Check sheet for the modelled part. Datum: model origin and axes. Units: mm. A direction names the side the tool comes from. Round coordinates to 2 decimals unless told otherwise and drop trailing zeros. Order: outer loops, then holes, each group sorted by start corner. A loop starts at its lowest first (then second) coordinate and runs counter-clockwise, first axis right, second up.
from build123d import *

# Parameters (mm, degrees)
SKETCH_1_R          = 14
SKETCH_1_R_2        = 7.5
EXTRUDE_1_DEPTH     = 35
SKETCH_2_R          = 7.5
CUT_EXTRUDE_1_DEPTH = 35
SKETCH_3_R          = 2.5
EXTRUDE_2_DEPTH     = 14
SKETCH_3_2_R        = 2.5
CUT_EXTRUDE_2_DEPTH = 3


with BuildPart() as part:
    # Sketch 1 → Extrude 1 (new body)
    with BuildSketch(Plane(origin=(0, 0, 0), x_dir=(1, 0, 0), z_dir=(0, 1, 0))):
        with Locations(Location((35, 0, 0), (0, 0, 270))):
            Circle(SKETCH_1_R)
        with Locations(Location((35, 0, 0), (0, 0, 270))):
            Circle(SKETCH_1_R_2, mode=Mode.SUBTRACT)
    extrude(amount=EXTRUDE_1_DEPTH)

    # Sketch 2 → Cut-Extrude 1 (cut)
    with BuildSketch(Plane.XY):
        with Locations(Location((35, 20, 0), (0, 0, 180))):
            Circle(SKETCH_2_R)
    extrude(amount=CUT_EXTRUDE_1_DEPTH, mode=Mode.SUBTRACT)

    # Sketch 3 → Extrude 2 (add)
    with BuildSketch(Plane.XY):
        Polygon((0, 0), (35, 0), (35, -7), (15, -7), (15, -18), (0, -18), align=None)
        with Locations((7, -13)):
            Circle(SKETCH_3_R, mode=Mode.SUBTRACT)
    extrude(amount=EXTRUDE_2_DEPTH)

    # Sketch 3_2 → Cut-Extrude 2 (cut)
    with BuildSketch(Plane.XY):
        Polygon((0, 0), (35, 0), (35, -7), (15, -7), (15, -18), (0, -18), align=None)
        with Locations((7, -13)):
            Circle(SKETCH_3_2_R, mode=Mode.SUBTRACT)
    extrude(amount=CUT_EXTRUDE_2_DEPTH, mode=Mode.SUBTRACT)


solid = part.part
1) Scan lines: line 1 (Y direction, x = 7, z = 9); line 2 (X direction, y = 12, z = 0); line 3 (Z direction, x = 5, y = -3). Record each from-to range of solid material in increasing order.
2) Sectioned sample at C-C on y = -13. Record the cut outline in (x, z), and give its area (3 significant figures).
3) Gauge pin test, flat ends, axial feed: pin 1 (2 mm diameter, centred on x = 32, z = 5, fed in from +Y); pin 2 (6 mm diameter, centred on y = 4.5, z = -3.5, fed in from +X); pin 3 (2 mm diameter, centred on x = 42, y = 24.5, fed in from +Z). Record the tip position at first contact, or that the pin passes through.
4) Sectioned sample at B-B on z = 3.75. Record the cut outline in (x, y).
5) Set-up check for faces 4 (the face through (13, 0, 8)), 5 (the face through (41, 0, -6)), 6 (the face through (35.33, 17.255, -7.493)): record each of +Z, -Z, +X, -X, +Y, -Y from which the full face is reachable in a straight line by a thin tool's end or side.
6) Sectioned sample at A-A on x = 8.5. Record the cut outline in (y, z), and give its area (3 significant figures).
7) Draft check along Z on faces 1 (the face through (35, -3, 8)), 2 (the face through (35.616, 17.255, -13.986)), 3 (the face through (32, 0, 5)). Enter one of: pulls with the +Z half, pulls with the -Z half, needs draft (parallel to the pull), parting line crosses it, or undercut.
8) Sectioned sample at D-D on z = 8.75. Record the cut outline in (x, y), and give its area (3 significant figures).
Values found:
1. line 1: y = -18 to -15.5, -10.5 to 0
1. line 2: x = 21 to 27.5, 42.5 to 49
1. line 3: z = 3 to 14
2. outline: (0, 3) - (4.5, 3) - (4.5, 14) - (0, 14) - close; (9.5, 3) - (15, 3) - (15, 14) - (9.5, 14) - close
2. area: 110 mm2
3. pin 1: stops at y = 0
3. pin 2: stops at x = 48.99
3. pin 3: stops at z = 12.65
4. outline: (0, -18) - (15, -18) - (15, -7) - (35, -7) - (35, 0) - (28.5, 0) - (28.5, 16.25) arc R7.5 cw to (28.5, 23.75) - (28.5, 35) - (21.51, 35) - (21.51, 0) - (0, 0) - close; (41.5, 0) - (48.49, 0) - (48.49, 35) - (41.5, 35) - (41.5, 23.75) arc R7.5 cw to (41.5, 16.25) - close; hole circle Ø5 at (7, -13)
5. face 4: +Z, -X, +Y
5. face 5: -Z, +X, -Y
5. face 6: +Y
6. outline: (-18, 3) - (-15, 3) - (-15, 14) - (-18, 14) - close; (-11, 3) - (0, 3) - (0, 14) - (-11, 14) - close
6. area: 154 mm2
7. face 1: needs draft
7. face 2: parting line crosses it
7. face 3: undercut
8. outline: (0, -18) - (15, -18) - (15, -7) - (35, -7) - (35, 0) - (45.93, 0) - (45.93, 35) - (24.07, 35) - (24.07, 0) - (0, 0) - close; hole circle Ø5 at (7, -13); hole circle Ø15 at (35, 20)
8. area: 979 mm2
